Input: part model. Units: mm. Frame: model coordinates. A direction names the side the tool comes from. Round coordinates to 2 decimals unless told otherwise and drop trailing zeros. Loops run counter-clockwise (first coordinate to the right, second up) from the corner with the lowest first, then second, coordinate; pieces in that order, holes last. Notation, with made-up numbers: (83, -16) -> (88, -16) arc R21 ccw to (88, 22) -> close; hole circle Ø5 at (-5, 81.25). An arc over 180 degrees is marked (long way). Answer as a JSON object with one key per item and string values. Group by question number.
Item 1: Draft query along X for faces 4 (the flat face through (17, 1, -26.7)), 5 (the flat face through (0, 1, -48.5)), 6 (the flat face through (7, 1, -47)). Return one class per face: released by +X, released by -X, zero draft, split by the parting line, or undercut.
Item 2: Material intervals for line 1 (X direction, y = 0.5, z = -33) (3 decimals); line 2 (X direction, y = 1.7, z = -38); line 3 (X direction, y = 0.2, z = -20.5), sorted ascending. Write a range as [from, to].
Item 3: Section query C-C on z = -23.5. Return loops of the section in (x, y).
Item 4: Section query D-D on x = -8.5. Return loops of the section in (y, z), and give its area (3 significant figures).
Item 5: Set-up query: faces 1 (the flat face through (15, 1, -45)), 2 (the flat face through (-15, 1, -45)), 3 (the cylindrical face through (11.579, 1.014, -7.246)). Return all of +Z, -Z, +X, -X, +Y, -Y with unobstructed straight access to the full face (end or side cutting, diameter ignored); none if empty.
Item 6: Pin query (flat end, axial travel): pin 1 (0.6 mm diameter, centred on y = 1.5, z = -46, fed in from -X); pin 2 (1 mm diameter, centred on x = 4.5, y = 0.5, fed in from +Z); pin 3 (1 mm diameter, centred on x = 16.5, y = 1, fed in from -Z). Return the tip coordinate at first contact, or that it passes through.
Item 7: Section query A-A on x = 0. Return loops of the section in (y, z) (3 decimals), and give its area (3 significant figures).
Item 8: Section query B-B on z = -18.5. Return loops of the section in (x, y), and give its area (3 significant figures).
from build123d import *

# Parameters (mm, degrees)
SKETCH1_R          = 1.5
EXTRUDE1_DEPTH     = 2
CUT_EXTRUDE1_DEPTH = 2
FILLET1_R          = 2
CUT_EXTRUDE3_REACH = 55.715
SKETCH3_R          = 1.5
SKETCH3_R_2        = 0.75
SKETCH3_R_3        = 2.5
CUT_EXTRUDE4_REACH = 55.715
FILLET2_R          = 0.5


with BuildPart() as part:
    # Sketch1 → Extrude1 (new body)
    with BuildSketch(Plane(origin=(0, 0, 0), x_dir=(1, 0, 0), z_dir=(0, 1, 0))):
        Polygon((-23, 0), (23, 0), (23, 45), (7, 45), (7, 48.5), (-7, 48.5), (-7, 45), (-23, 45), align=None)
        with Locations(Location((-18.5, 6, 0), (0, 0, 270))):
            Circle(SKETCH1_R, mode=Mode.SUBTRACT)
        with Locations(Location((18.5, 18.5, 0), (0, 0, 270))):
            Circle(SKETCH1_R, mode=Mode.SUBTRACT)
    extrude(amount=EXTRUDE1_DEPTH)

    # Sketch2 → Cut-Extrude1 (cut)
    with BuildSketch(Plane(origin=(0, 2, 0), x_dir=(1, 0, 0), z_dir=(0, 1, 0))):
        with BuildLine():
            Line((-5.95, 4.95), (5.95, 4.95))
            ThreePointArc((5.95, 4.95), (11.642209589, 7.307790411), (14, 13))
            Line((14, 13), (14, 32.9))
            Line((14, 32.9), (-14, 32.9))
            Line((-14, 32.9), (-14, 13))
            ThreePointArc((-14, 13), (-11.642209589, 7.307790411), (-5.95, 4.95))
        make_face()
    extrude(amount=-CUT_EXTRUDE1_DEPTH, mode=Mode.SUBTRACT)

    # Fillet1
    fillet1_edges = [part.edges().sort_by_distance(p)[0] for p in [
        (-14, 1, -32.9),
        (14, 1, -32.9),
    ]]
    fillet(fillet1_edges, radius=FILLET1_R)

    # Sketch3 → Cut-Extrude3 (cut, up to next)
    with BuildSketch(Plane(origin=(0, 2, 0), x_dir=(1, 0, 0), z_dir=(0, 1, 0)), mode=Mode.PRIVATE) as cut_extrude3_sk1:
        with Locations(Location((0, 45.257858412, 0), (0, 0, 270))):
            Circle(SKETCH3_R)
    cut_extrude3_tool1 = extrude(cut_extrude3_sk1.sketch, amount=-CUT_EXTRUDE3_REACH, mode=Mode.PRIVATE) & part.part
    # Sketch3 → Cut-Extrude3 (cut, up to next)
    with BuildSketch(Plane(origin=(0, 2, 0), x_dir=(1, 0, 0), z_dir=(0, 1, 0)), mode=Mode.PRIVATE) as cut_extrude3_sk2:
        with Locations(Location((-19.625, 33, 0), (0, 0, 270))):
            Circle(SKETCH3_R_2)
    cut_extrude3_tool2 = extrude(cut_extrude3_sk2.sketch, amount=-CUT_EXTRUDE3_REACH, mode=Mode.PRIVATE) & part.part
    # Sketch3 → Cut-Extrude3 (cut, up to next)
    with BuildSketch(Plane(origin=(0, 2, 0), x_dir=(1, 0, 0), z_dir=(0, 1, 0)), mode=Mode.PRIVATE) as cut_extrude3_sk3:
        with Locations(Location((19.625, 33, 0), (0, 0, 270))):
            Circle(SKETCH3_R_2)
    cut_extrude3_tool3 = extrude(cut_extrude3_sk3.sketch, amount=-CUT_EXTRUDE3_REACH, mode=Mode.PRIVATE) & part.part
    # Sketch3 → Cut-Extrude3 (cut, up to next)
    with BuildSketch(Plane(origin=(0, 2, 0), x_dir=(1, 0, 0), z_dir=(0, 1, 0)), mode=Mode.PRIVATE) as cut_extrude3_sk4:
        with Locations(Location((0, 37.925, 0), (0, 0, 270))):
            Circle(SKETCH3_R_3)
    cut_extrude3_tool4 = extrude(cut_extrude3_sk4.sketch, amount=-CUT_EXTRUDE3_REACH, mode=Mode.PRIVATE) & part.part
    add(cut_extrude3_tool1.solids().sort_by_distance((0, 2, -45.257858))[0], mode=Mode.SUBTRACT)
    add(cut_extrude3_tool2.solids().sort_by_distance((-19.625, 2, -33))[0], mode=Mode.SUBTRACT)
    add(cut_extrude3_tool3.solids().sort_by_distance((19.625, 2, -33))[0], mode=Mode.SUBTRACT)
    add(cut_extrude3_tool4.solids().sort_by_distance((0, 2, -37.925))[0], mode=Mode.SUBTRACT)

    # Sketch10 → Cut-Extrude4 (cut, up to next)
    with BuildSketch(Plane(origin=(0, 2, 0), x_dir=(1, 0, 0), z_dir=(0, 1, 0)), mode=Mode.PRIVATE) as cut_extrude4_sk1:
        Polygon((14, 26.7), (19.8, 26.7), (19.8, 28.5), (16.3, 28.5), (16.3, 28), (14, 28), align=None)
    cut_extrude4_tool1 = extrude(cut_extrude4_sk1.sketch, amount=-CUT_EXTRUDE4_REACH, mode=Mode.PRIVATE) & part.part
    add(cut_extrude4_tool1.solids().sort_by_distance((17.116631, 2, -27.519537))[0], mode=Mode.SUBTRACT)

    # Fillet2
    fillet2_edges = [part.edges().sort_by_distance(p)[0] for p in [
        (16.3, 1, -28.5),
        (19.8, 1, -28.5),
        (19.8, 1, -26.7),
        (14, 1, -28),
        (14, 1, -26.7),
    ]]
    fillet(fillet2_edges, radius=FILLET2_R - 0.0001)  # a hair under: the kernel refuses the full size


solid = part.part
Solved:
{
 "1": {"face 4": "undercut", "face 5": "zero draft", "face 6": "released by +X"},
 "2": {"line 1": "[-23, -20.375], [-18.875, 18.875], [20.375, 23]", "line 2": "[-23, -2.5], [2.5, 23]", "line 3": "[-23, -14], [14, 23]"},
 "3": {"outline": "(-23, 0) -> (-14, 0) -> (-14, 2) -> (-23, 2) -> close; (14, 0) -> (23, 0) -> (23, 2) -> (14, 2) -> close"},
 "4": {"outline": "(0, -45) -> (2, -45) -> (2, -32.9) -> (0, -32.9) -> close; (0, -5.36) -> (2, -5.36) -> (2, 0) -> (0, 0) -> close", "area": "34.9 mm²"},
 "5": {"face 1": "-Z, +X, +Y, -Y", "face 2": "-Z, -X, +Y, -Y", "face 3": "+Y, -Y"},
 "6": {"pin 1": "x = -7", "pin 2": "z = 0", "pin 3": "z = -45"},
 "7": {"outline": "(0, -48.5) -> (2, -48.5) -> (2, -46.758) -> (0, -46.758) -> close; (0, -43.758) -> (2, -43.758) -> (2, -40.425) -> (0, -40.425) -> close; (0, -35.425) -> (2, -35.425) -> (2, -32.9) -> (0, -32.9) -> close; (0, -4.95) -> (2, -4.95) -> (2, 0) -> (0, 0) -> close", "area": "25.1 mm²"},
 "8": {"outline": "(-23, 0) -> (-14, 0) -> (-14, 2) -> (-23, 2) -> close; (14, 0) -> (17, 0) -> (17, 2) -> (14, 2) -> close; (20, 0) -> (23, 0) -> (23, 2) -> (20, 2) -> close", "area": "30.0 mm²"}
}
